```python
from build123d import *

# Parameters (mm, degrees)
BOSS_EXTRUDE1_DEPTH      = 6.35
CUT_EXTRUDE2_DEPTH       = 7.3500001
SKETCH8_W                = 698.5
SKETCH8_H                = 57.15
BOSS_EXTRUDE3_DEPTH      = 6.35
SKETCH12_W               = 58.7375
SKETCH12_H               = 57.15
CUT_EXTRUDE3_DEPTH       = 7.3500001
FILLET2_R                = 3.175
FILLET3_R                = 6.35
F_0_257_DIAMETER_HOLE2_D = 6.5278


with BuildPart() as part:
    # Sketch1 → Boss-Extrude1 (new body)
    with BuildSketch(Plane.XY):
        with BuildLine():
            Line((0, 254), (0, 0))
            Line((0, 0), (1092.2, 0))
            add(Edge.make_bspline(
                [(0, 254), (376.513153864, 252.276375478), (770.285770075, 140.499670678), (1092.2, 0)],
                knots=[0, 0, 0, 0, 1, 1, 1, 1], degree=3))
        make_face()
    extrude(amount=BOSS_EXTRUDE1_DEPTH)

    # Sketch7 → Cut-Extrude2 (cut, through all)
    with BuildSketch(Plane(origin=(0, 0, 0), x_dir=(-1, 0, 0), z_dir=(0, 0, -1))):
        with BuildLine():
            Line((-133.35, 0), (-63.5, 0))
            ThreePointArc((-63.5, 0), (-65.359871939, 4.490128061), (-69.85, 6.35))
            Line((-69.85, 6.35), (-133.35, 6.35))
            ThreePointArc((-133.35, 6.35), (-137.840128061, 4.490128061), (-139.7, 0))
            Line((-139.7, 0), (-133.35, 0))
        make_face()
    extrude(amount=-CUT_EXTRUDE2_DEPTH, mode=Mode.SUBTRACT)

    # Sketch8 → Boss-Extrude3 (add)
    with BuildSketch(Plane.XY.offset(6.35)):
        with Locations((541.3375, -28.575)):
            Rectangle(SKETCH8_W, SKETCH8_H)
    extrude(amount=-BOSS_EXTRUDE3_DEPTH)

    # Sketch12 → Cut-Extrude3 (cut, through all)
    with BuildSketch(Plane.XY.offset(6.35)):
        with Locations((575.46875, -28.575)):
            Rectangle(SKETCH12_W, SKETCH12_H)
    extrude(amount=-CUT_EXTRUDE3_DEPTH, mode=Mode.SUBTRACT)

    # Fillet2
    fillet2_edges = [part.edges().sort_by_distance(p)[0] for p in [
        (192.0875, 0, 3.175),
        (890.5875, 0, 3.175),
        (604.8375, 0, 3.175),
        (546.1, 0, 3.175),
    ]]
    fillet(fillet2_edges, radius=FILLET2_R)

    # Fillet3
    fillet3_edges = [part.edges().sort_by_distance(p)[0] for p in [
        (192.0875, -57.15, 3.175),
        (890.5875, -57.15, 3.175),
        (604.8375, -57.15, 3.175),
        (546.1, -57.15, 3.175),
    ]]
    fillet(fillet3_edges, radius=FILLET3_R)

    # F (0.257) Diameter Hole2 (through all)
    with Locations(Plane(origin=(0, 0, 0), x_dir=(-1, 0, 0), z_dir=(0, 0, -1))):
        with Locations((-847.725, -35.306), (-234.95, -35.306)):
            Hole(F_0_257_DIAMETER_HOLE2_D / 2)


solid = part.part
```
Source: CAD feature listing. Evaluate the final solid. Frame: model axes, mm. Give positions to 0.01 mm unless a question says otherwise; leave off trailing zeros.
1. First-contact query: pin 1 (1.9 mm diameter, centred on x = 28.5, z = 2, fed in from -Y); pin 2 (3 mm diameter, centred on y = -24, z = 4, fed in from -X); pin 3 (8.5 mm diameter, centred on x = 234.95, y = -35.306, fed in from +Z). Flat tips, straight axial feed; report the tip coordinate or a pass-through.
2. Section query A-A (z = 3.25). Count the separate pieces of the cut face and the enclosed holes in it, then the cut area to 3 significant figures.
3. Material intervals for line 1 along Y through (x, z) = (234.95, 4.5); line 2 along Y through (x, z) = (370.5, 1.5); line 3 along Y through (x, z) = (1021, 3.75), sorted ascending.
Output values:
1. pin 1: stops at y = 0
1. pin 2: stops at x = 192.09
1. pin 3: stops at z = 6.35
2. separate pieces: 1
2. enclosed holes: 2
2. area: 216,000 mm2
3. line 1: y = -57.15 to -38.57, -32.04 to 239.54
3. line 2: y = -57.15 to 220.07
3. line 3: y = 0 to 30.11
